Can you work these out from the model? Positions are in its coordinate system, mm. Face numbers are marked on the shaded views. A direction names the side the tool comes from. Coordinates: 2 decimals unless noted, no trailing zeros. Write each loop counter-clockwise with the first axis right and the second up, starting at its lowest first coordinate (ties: lowest second). Pieces come first, ordered by that corner, then holes.
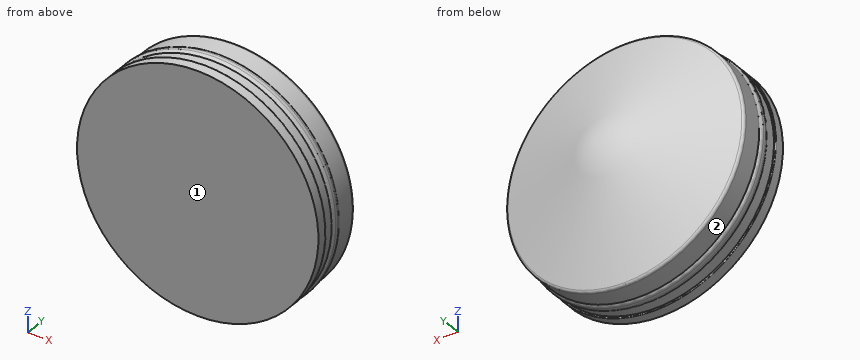
```python
from build123d import *

# Parameters (mm, degrees)
SKETCH1_R           = 11.25
BOSS_EXTRUDE1_DEPTH = 1
SKETCH2_R           = 11.105
BOSS_EXTRUDE2_DEPTH = 1
SKETCH3_R           = 11.25
BOSS_EXTRUDE3_DEPTH = 1
SKETCH4_R           = 11.1
BOSS_EXTRUDE4_DEPTH = 2
FILLET1_R           = 0.3
FILLET3_R           = 0.5
FILLET4_R           = 0.06


with BuildPart() as part:
    # Sketch1 → Boss-Extrude1 (new body)
    with BuildSketch(Plane(origin=(0, 0, 0), x_dir=(1, 0, 0), z_dir=(0, 1, 0))):
        with Locations(Location((0, 0, 0), (0, 0, 270))):
            Circle(SKETCH1_R)
    extrude(amount=BOSS_EXTRUDE1_DEPTH)

    # Sketch2 → Boss-Extrude2 (add)
    with BuildSketch(Plane(origin=(0, 1, 0), x_dir=(1, 0, 0), z_dir=(0, 1, 0))):
        with Locations(Location((0, 0, 0), (0, 0, 270))):
            Circle(SKETCH2_R)
    extrude(amount=BOSS_EXTRUDE2_DEPTH)

    # Sketch3 → Boss-Extrude3 (add)
    with BuildSketch(Plane(origin=(0, 2, 0), x_dir=(1, 0, 0), z_dir=(0, 1, 0))):
        with Locations(Location((0, 0, 0), (0, 0, 270))):
            Circle(SKETCH3_R)
    extrude(amount=BOSS_EXTRUDE3_DEPTH)

    # Sketch4 → Boss-Extrude4 (add)
    with BuildSketch(Plane(origin=(0, 3, 0), x_dir=(1, 0, 0), z_dir=(0, 1, 0))):
        with Locations(Location((0, 0, 0), (0, 0, 270))):
            Circle(SKETCH4_R)
    extrude(amount=BOSS_EXTRUDE4_DEPTH)

    # Sketch6 → Revolve1 (revolve)
    with BuildSketch(Plane(origin=(0, 0, 0), x_dir=(0.06000839273320703, 0, 0.9981978725691502), z_dir=(-0.9981978725691503, 0, 0.06000839273320704)), mode=Mode.PRIVATE) as revolve1_sk:
        Polygon((11.1, 5), (0, 5), (0, 9), align=None)
    revolve(revolve1_sk.sketch.rotate(Axis((0, 5, 0), (0, 1, 0)), 176.559705496), axis=Axis((0, 5, 0), (0, 1, 0)))

    # Fillet1
    fillet1_edges = [part.edges().sort_by_distance(p)[0] for p in [
        (-11.1, 5, 0),
    ]]
    fillet(fillet1_edges, radius=FILLET1_R)

    # Fillet3
    # the kernel refuses this fillet: 0.5 mm, written as the material it takes off along each edge
    with BuildSketch(Plane(origin=(0, 3, 0), x_dir=(0, 0, 1), z_dir=(-1, 0, 0))) as fillet3_piece_1:
        with BuildLine():
            CenterArc((10.75, -0.357071421), FILLET3_R, 0, 45.572995999)
            Line((11.25, -0.357071421), (11.26, -0.357071421))
            Line((11.26, -0.357071421), (11.26, 0))
            Line((11.26, 0), (11.25, 0.01))
            ThreePointArc((11.25, 0.01), (11.175, 0.01), (11.107, 0.007141428))
            Line((11.107, 0.007141428), (11.1, 0))
        make_face()
    revolve(axis=Axis((0, 3, 0), (0, 1, 0)), mode=Mode.SUBTRACT)
    with BuildSketch(Plane(origin=(0, 2, 0), x_dir=(0, 0, 1), z_dir=(-1, 0, 0))) as fillet3_piece_2:
        with BuildLine():
            CenterArc((10.75, 0.352100838), FILLET3_R, 315.234915329, 44.765084671)
            Line((11.105, 0), (11.1121, -0.007042017))
            ThreePointArc((11.1121, -0.007042017), (11.1775, -0.01), (11.25, -0.01))
            Line((11.25, -0.01), (11.26, 0))
            Line((11.26, 0), (11.26, 0.352100838))
            Line((11.26, 0.352100838), (11.25, 0.352100838))
        make_face()
    revolve(axis=Axis((0, 2, 0), (0, 1, 0)), mode=Mode.SUBTRACT)

    # Fillet4
    fillet4_edges = [part.edges().sort_by_distance(p)[0] for p in [
        (0, 1, -11.25),
    ]]
    fillet(fillet4_edges, radius=FILLET4_R)


solid = part.part
```
1. Which directions (+Z, -Z, +X, -X, +Y, -Y) give clear straight access to the entire face, cutting with the end or side of a thin tool? Please do the marked faces 1 and 2.
2. If I drill on L1, parallel to X at y = 4, z = -1.25; L2, parallel to Y at x = -6, z = -1.25; L3, parallel to Y at x = 3.5, z = -4, over which ranges is the centre line in solid material (lowest first)?
3. I'm going to push flat-ended pins straight in: P1, Ø2, axis at y = 1.5, z = -2.5, coming from the -X side; P2, Ø5, axis at y = 5.5, z = 1.5, coming from the +X side; P3, Ø1.5, axis at x = 8, z = 5, coming from the +Y side. Where does each tip first touch, or does it pass through?
4. If we section it at B-B, the plane y = 6.25: List the corners of the cut face in (x, z) for me, plus the area to 3 significant figures.
5. If we section it at A-A, the plane y = 7.5: List the corners of the cut face in (x, z) for me (1 decimal).
Answers:
1. face 1: +Z, -Z, +X, -X, -Y
1. face 2: +Y
2. L1: x = -11.03 to 11.03
2. L2: y = 0 to 6.79
2. L3: y = 0 to 7.08
3. P1: stops at x = -11.13
3. P2: stops at x = 11.1
3. P3: stops at y = 5.87
4. outline: circle Ø15.26 at (0, 0)
4. area: 183 mm2
5. outline: circle Ø8.3 at (0, 0)
